For this review, take the finished solid that the model builds, in its own axes (mm). A direction names the side the tool comes from. Coordinates: 2 decimals unless noted, no trailing zeros. Loops run counter-clockwise (first coordinate to the right, second up) from the corner with the lowest first, then second, coordinate; pieces in that order, holes last.
1. Take a section at A-A, the plane x = 0. State the section outline as (y, z) points.
2. Take a section at D-D, the plane z = 18.5. State the section outline as (x, y) points, then the cut area to 3 significant figures.
3. Take a section at C-C, the plane y = -3.5. State the section outline as (x, z) points.
4. Mouldability with a two-part tool opening along X and no side actions: class faces 5 (the face through (0, -3, 52)), 6 (the face through (-0.26, -0.042, 56.483)), 7 (the face through (-4.384, -0.045, 53.96)), 8 (the face through (0, 0, 59)) as pulls with the +X half, pulls with the -X half, needs draft (parallel to the pull), parting line crosses it, or undercut.
5. To check wall thickness, follow probe 1 along Z at (x, y) = (0, -1.8); probe 2 along X at (y, z) = (-3, 6); probe 3 along X at (y, z) = (1, 44). State the ranges of each line that lie inside material, in increasing order.
6. Clearance check with flat-ended pins moving along their axes: P1, Ø3, axis at x = -3, y = -0.5, coming from the +Z side; P2, Ø1.5, axis at y = 1.5, z = 10, coming from the +X side; P3, Ø1.3, axis at x = -4, y = 0.5, coming from the +Z side. State where each tip first meets the part, or that it passes through.
7. Take a section at B-B, the plane z = 54.5. State the section outline as (x, y) points.
8. Machinability: for faces 1 (the face through (4.384, 0.045, 53.96)), 2 (the face through (0, -4, 50)), 3 (the face through (-0.59, -4.46, 24.65)), 4 (the face through (0, 3, 52)), which of the approach directions +Z, -Z, +X, -X, +Y, -Y give a long, thin tool a straight path to every point of the face, cutting with its end or side? Answer none if there is none.
Autodesk Inventor part; units mm, degrees
ref_plane "YZ Plane" through (0, 0, 0) normal (1, 0, 0) x (0, 1, 0)
ref_plane "XZ Plane" through (0, 0, 0) normal (0, 1, 0) x (-1, 0, 0)
ref_plane "XY Plane" through (0, 0, 0) normal (0, 0, 1) x (1, 0, 0)
sketch "Sketch1" plane through (0, 0, 0) normal (0, 0, 1) x (1, 0, 0)
  circle A0 centre (0, 0) radius 4.5
  dimension "d0" = 9
extrude "Extrusion1" add sketch "Sketch1" along normal blind 50
sketch "Sketch2" plane through (0, 0, 50) normal (0, 0, 1) x (1, 0, 0)
  circle A0 centre (0, 0) radius 4.5
  line L0 (-3.3541, 3) -> (3.3541, 3)
  line L1 (3.3541, 3) -> (3.3541, -3)
  line L2 (3.3541, -3) -> (-3.3541, -3)
  line L3 (-3.3541, -3) -> (-3.3541, 3)
  circle A1 centre (0, 0) radius 4.5
  line L4 (-4.5, 0) -> (4.5, 0) construction
  arc A2 (-3.3541, 3) -> (-3.3541, -3) centre (0.5, 0) ccw
  line L5 (0, 3) -> (0, -3) construction
  arc A3 (3.3541, -3) -> (3.3541, 3) centre (-0.5, 0) ccw
  point P0 (-3.3541, 0)
  dimension "d3" = 6
  dimension "d4" = 0.5
extrude "Extrusion2" add sketch "Sketch2" along normal blind 9 contours L1 L2 L3 L0 | A3 L1 | L3 A2
sketch "Sketch3" plane through (-3.3541, -3, 50) normal (0, -1, 0) x (1, 0, 0)
  line L0 (7.7382, 0) -> (7.7382, 9)
  line L1 (-1.03, 0) -> (-1.03, 9)
  arc A0 (7.7382, 8) -> (-1.03, 8) centre (3.3541, -1.11) ccw
  line L2 (0, 9) -> (6.7082, 9)
  line L3 (0, 9) -> (-1.03, 9)
  line L4 (7.7382, 9) -> (6.7082, 9)
  point P0 (3.3541, -50)
  point P1 (3.3541, 9)
  dimension "d7" = 1
  dimension "d8" = 1
extrude "Extrusion3" cut sketch "Sketch3" against normal through all
fillet "Fillet1" radius 0.5 4 edges at (-4.1284, -1.5596, 58.1187) (-4.1284, 1.5596, 58.1187) (4.1284, 1.5596, 58.1187) (4.1284, -1.5596, 58.1187)
sketch "Sketch4" plane through (-3.3541, -3, 50) normal (0, -1, 0) x (1, 0, 0)
  line L0 (6.7082, 0) -> (0, 0) construction
  line L1 (3.3541, 0) -> (3.3541, 9) construction
  arc A0 (6.1913, 8.5937) -> (0.5169, 8.5937) centre (3.3541, -1.11) ccw construction
  circle A1 centre (3.3541, 4.5) radius 2
  line L2 (0, 0) -> (0, 8.0329)
  line L3 (0, 6.5) -> (6.7082, 6.5) construction
  line L4 (6.7082, 0) -> (6.7082, 8.0329)
  point P0 (3.3541, -50)
  point P1 (3.3541, 9)
  dimension "d12" = 4
  dimension "d13" = 2.5
extrude "Extrusion4" cut sketch "Sketch4" against normal through all
properties part number "LA-T8-1215-50 105-64 Shaft"
Results list:
1. outline: (-4.5, 0) - (4.5, 0) - (4.5, 50) - (3, 50) - (3, 52.5) - (-3, 52.5) - (-3, 50) - (-4.5, 50) - close; (-3, 56.5) - (3, 56.5) - (3, 59) - (-3, 59) - close
2. outline: circle Ø9 at (0, 0)
2. area: 63.6 mm2
3. outline: (-2.83, 0) - (2.83, 0) - (2.83, 50) - (-2.83, 50) - close
4. face 5: needs draft
4. face 6: undercut
4. face 7: pulls with the -X half
4. face 8: parting line crosses it
5. probe 1: z = 0 to 52.5, 56.5 to 59
5. probe 2: x = -3.35 to 3.35
5. probe 3: x = -4.39 to 4.39
6. P1: stops at z = 58.89
6. P2: stops at x = 4.44
6. P3: stops at z = 58.43
7. outline: (-3.35, -3) - (-2, -3) - (-2, 3) - (-3.35, 3) arc R4.88 ccw to start; (2, -3) - (3.35, -3) arc R4.88 ccw to (3.35, 3) - (2, 3) - close
8. face 1: +Z, +X
8. face 2: +Z, +X, -X, -Y
8. face 3: +Z, -Z
8. face 4: +Z, +X, -X, +Y
